The model under review builds one solid part; all positions refer to its coordinate system, in mm. Coordinates: 2 decimals unless noted, no trailing zeros. Order: outer loops, then holes, each group sorted by start corner. A loop starts at its lowest first (then second) coordinate and runs counter-clockwise, first axis right, second up. Notation, with made-up numbers: (24.5, 27) -> (66.5, 27) arc R26 cw to (66.5, 49) -> close; hole circle Ø11 at (24.5, 24). An arc over 180 degrees is marked (long way). Put each result on its own line as item: value.
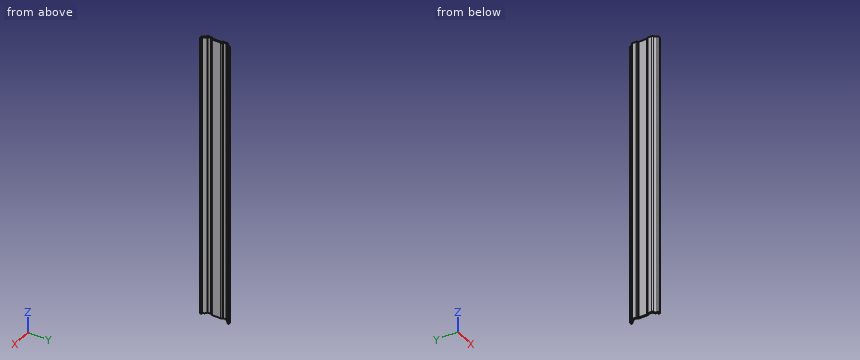
from build123d import *

# Parameters (mm, degrees)
EXTRUDE_THIN1_DEPTH = 357.1875
FILLET1_R           = 1.651


with BuildPart() as part:
    # Sketch1 → Extrude-Thin1 (new body)
    with BuildSketch(Plane.XY):
        with BuildLine():
            Line((0, 0), (-3.697192387, 0))
            ThreePointArc((-3.697192387, 0), (-4.204355265, 3.261336848), (-7.14375, 4.7625))
            Line((-7.14375, 4.7625), (-7.14375, 11.1125))
            Line((-7.14375, 11.1125), (-5.715, 12.668334975))
            Line((-5.715, 12.668334975), (-5.715, 23.050415025))
            Line((-5.715, 23.050415025), (-7.14375, 24.60625))
            Line((-7.14375, 24.60625), (-7.14375, 30.95625))
            ThreePointArc((-7.14375, 30.95625), (-4.204355265, 32.457413152), (-3.697192387, 35.71875))
            Line((-3.697192387, 35.71875), (0, 35.71875))
            Line((0, 35.71875), (0, 34.06775))
            Line((0, 34.06775), (-1.889748251, 34.06775))
            ThreePointArc((-1.889748251, 34.06775), (-3.02342288, 31.283918913), (-5.49275, 29.570046904))
            Line((-5.49275, 29.570046904), (-5.49275, 25.249313927))
            Line((-5.49275, 25.249313927), (-4.064, 23.693478952))
            Line((-4.064, 23.693478952), (-4.064, 12.025271048))
            Line((-4.064, 12.025271048), (-5.49275, 10.469436073))
            Line((-5.49275, 10.469436073), (-5.49275, 6.148703096))
            ThreePointArc((-5.49275, 6.148703096), (-3.02342288, 4.434831087), (-1.889748251, 1.651))
            Line((-1.889748251, 1.651), (0, 1.651))
            Line((0, 1.651), (0, 0))
        make_face()
    extrude(amount=-EXTRUDE_THIN1_DEPTH)

    # Fillet1
    fillet1_edges = [part.edges().sort_by_distance(p)[0] for p in [
        (-3.697192387, 0, -178.59375),
        (-7.14375, 4.7625, -178.59375),
        (-7.14375, 11.1125, -178.59375),
        (-7.14375, 24.60625, -178.59375),
        (-7.14375, 30.95625, -178.59375),
        (-3.697192387, 35.71875, -178.59375),
        (-4.064, 23.693478952, -178.59375),
        (-4.064, 12.025271048, -178.59375),
    ]]
    fillet(fillet1_edges, radius=FILLET1_R)


solid = part.part
Item 1: For pin 1 Ø5 at (y, z) = (30, -36) entering from +X; pin 2 Ø4 at (y, z) = (11, -191.5) entering from +X; pin 3 Ø2 at (x, z) = (-1.5, -259.5) entering from -Y; pin 4 Ø1.3 at (y, z) = (9, -124) entering from +X, all flat-tipped, find the tip position at first contact; note any pin that passes through.
Answers below:
pin 1: x = -2.29
pin 2: x = -4.06
pin 3: y = 0
pin 4: x = -5.49
Item 2: For line 1 (Y direction, x = -1, z = -243.5); line 2 (X direction, y = 29.5, z = -150); line 3 (Y direction, x = -4.25, z = -266.5), list the stretches that pass through material, from the lowest coordinate up. Write a range as from..to.
Answers below:
line 1: 0..1.65, 34.07..35.72
line 2: -7.14..-5.49
line 3: 3.32..5.55, 11.91..23.81, 30.17..32.4
Item 3: Consider section A-A on z = -192. Write out the cut boundary in (x, y) (3 decimals).
Answers below:
outline: (-7.144, 6.149) arc R1.651 ccw to (-6.009, 4.581) arc R3.628 cw to (-3.533, 1.489) arc R1.651 ccw to (-1.89, 0) -> (0, 0) -> (0, 1.651) -> (-1.89, 1.651) arc R5.279 ccw to (-5.493, 6.149) -> (-5.493, 10.469) -> (-4.499, 11.552) arc R1.651 ccw to (-4.064, 12.668) -> (-4.064, 23.05) arc R1.651 ccw to (-4.499, 24.167) -> (-5.493, 25.249) -> (-5.493, 29.57) arc R5.279 ccw to (-1.89, 34.068) -> (0, 34.068) -> (0, 35.719) -> (-1.89, 35.719) arc R1.651 ccw to (-3.533, 34.229) arc R3.628 cw to (-6.009, 31.138) arc R1.651 ccw to (-7.144, 29.57) -> (-7.144, 25.249) arc R1.651 ccw to (-6.709, 24.133) -> (-5.715, 23.05) -> (-5.715, 12.668) -> (-6.709, 11.586) arc R1.651 ccw to (-7.144, 10.469) -> close
Item 4: Consider section B-B on y = 16. Write out the cut boundary in (x, z) (1 decimal), and give its area (3 significant figures).
Answers below:
outline: (-5.7, -357.2) -> (-4.1, -357.2) -> (-4.1, 0) -> (-5.7, 0) -> close
area: 590 mm^2
